Geometry check sheet. Reference: the model listing, model coordinates, mm. A direction names the side the tool comes from. Coordinates: 2 decimals unless noted, no trailing zeros. Write each loop counter-clockwise with the first axis right and the second up, starting at its lowest first coordinate (ties: lowest second). Pieces come first, ordered by that corner, then holes. Notation, with made-up numbers: (-36.5, 65) -> (8.5, 65) arc R19 cw to (8.5, 87) -> close; hole circle Ø5 at (1, 50.5). An arc over 180 degrees is marked (long way). Use a Markdown table: item, result.
```python
from build123d import *

# Parameters (mm, degrees)
F3_DEPTH = 0.2
F4_COUNT = 4
F7_DEPTH = 0.2


with BuildPart() as f1:
    # F0 (on Front) → F1 (revolve)
    with BuildSketch(Plane.XZ):
        with BuildLine():
            Line((0, 20.1388888889), (0, 0))
            Line((0, 0), (0.5555555556, 0))
            Line((0.5555555556, 0), (0.5555555556, 18.9583333333))
            Line((0.5555555556, 18.9583333333), (0.4513888889, 19.7916666667))
            ThreePointArc((0.4513888889, 19.7916666667), (0.2847433935, 20.0420414116), (0, 20.1388888889))
        make_face()
    revolve(axis=Axis((0, 0, 10.0694444444), (0, 0, 1)))

    # F2 (on Front) → F3 (join, symmetric)
    with BuildSketch(Plane.XZ):
        Polygon((0.2263558201, 19.9583333333), (-0.2263558201, 19.9583333333), (-1.8229166667, 17.9861111111), (-0.4993386243, 17.9861111111), (-2.3263888889, 15.7291666667), (2.3263888889, 15.7291666667), (0.4993386243, 17.9861111111), (1.8229166667, 17.9861111111), align=None)
        Polygon((0.5361597759, 0.0173323988), (0.5555555556, 0), (2.1875, -1.4583333333), (2.1875, 0.6597222222), (1.0069444444, 2.8125), (0.7291666667, 9.2361111111), (-0.7291666667, 9.2361111111), (-1.0069444444, 2.8125), (-2.1875, 0.6597222222), (-2.1875, -1.4583333333), (-0.5555555556, 0), (-0.5361597759, 0.0173323988), align=None)
        Polygon((-0.5555555556, 0), (0.5555555556, 0), (0.5361597759, 0.0173323988), (-0.5361597759, 0.0173323988), align=None)
    extrude(amount=F3_DEPTH, both=True)


with BuildPart() as f4_1:
    # F4: instance of F1
    add(f1.part.rotate(Axis((0, 0, 0), (0, 0, 1)), 1 * 360 / F4_COUNT))


with BuildPart() as f4_2:
    # F4: instance of F1
    add(f1.part.rotate(Axis((0, 0, 0), (0, 0, 1)), 2 * 360 / F4_COUNT))


with BuildPart() as f4_3:
    # F4: instance of F1
    add(f1.part.rotate(Axis((0, 0, 0), (0, 0, 1)), 3 * 360 / F4_COUNT))


with BuildPart() as f1_1:
    add(f1.part)

    add(f4_1.part)  # F7 merges F4_1

    add(f4_2.part)  # F7 merges F4_2

    add(f4_3.part)  # F7 merges F4_3
    # F6 (on face) → F7 (join, symmetric)
    with BuildSketch(Plane(origin=(0, 0, 0), x_dir=(0.7071067812, -0.7071067812, 0), z_dir=(-0.7071067812, -0.7071067812, 0))):
        Polygon((0.25, 15.3652419184), (-0.25, 15.3652419184), (-1.4370362347, 15), (-1.4370362347, 14.6875), (-0.25, 15.0527419184), (0.25, 15.0527419184), (1.4370362347, 14.6875), (1.4370362347, 15), align=None)
    extrude(amount=F7_DEPTH, both=True)


solid = f1_1.part
```
Item 1: Depth check by flat-ended pin: P1, Ø0.9, axis at x = 1.5, z = 17, coming from the +Y side; P2, Ø0.9, axis at y = -1.5, z = 16.5, coming from the +X side; P3, Ø1.4, axis at y = 1.5, z = 17, coming from the -X side. Enter the tip coordinate at first touch or a pass-through.
Answer block:
| item | result |
|---|---|
| P1 | stops at y = 0.2 |
| P2 | stops at x = 0.2 |
| P3 | stops at x = -0.2 |
Item 2: Section check D-D on x = 0. Record the boundary of the cut face in (y, z), then the cut area to 3 significant figures.
Answer block:
| item | result |
|---|---|
| outline | (-2.33, 15.73) -> (-0.56, 15.73) -> (-0.56, 9.24) -> (-0.73, 9.24) -> (-1.01, 2.81) -> (-2.19, 0.66) -> (-2.19, -1.46) -> (-0.56, 0) -> (0.56, 0) -> (2.19, -1.46) -> (2.19, 0.66) -> (1.01, 2.81) -> (0.73, 9.24) -> (0.56, 9.24) -> (0.56, 15.73) -> (2.33, 15.73) -> (0.56, 17.92) -> (0.56, 17.99) -> (1.82, 17.99) -> (0.47, 19.66) -> (0.45, 19.79) arc R0.47 ccw to (-0.45, 19.79) -> (-0.47, 19.66) -> (-1.82, 17.99) -> (-0.56, 17.99) -> (-0.56, 17.92) -> close |
| area | 41.1 mm^2 |
Item 3: Thickness scan on L1, parallel to Y at x = -1, z = 0.25; L2, parallel to Z at x = -1.9, y = 0.05. Record the ranges inside material, lowest first. Write a range as [from, to].
Answer block:
| item | result |
|---|---|
| L1 | y = [-0.2, 0.2] |
| L2 | z = [-1.2, 1.18], [15.73, 16.26] |
Item 4: Section check B-B on y = 1.45. Record the boundary of the cut face in (x, z), then the cut area to 3 significant figures.
Answer block:
| item | result |
|---|---|
| outline | (-0.2, -0.8) -> (0.2, -0.8) -> (0.2, 2) -> (-0.2, 2) -> close; (-0.2, 15.73) -> (0.2, 15.73) -> (0.2, 16.81) -> (-0.2, 16.81) -> close; (-0.2, 17.99) -> (0.2, 17.99) -> (0.2, 18.45) -> (-0.2, 18.45) -> close |
| area | 1.74 mm^2 |
Item 5: Tool access check on faces 1 (the flat face through (-1.383, -0.003, -0.739)), 2 (the flat face through (1.605, -0.003, 1.721)), 3 (the flat face through (0.8, 0.2, 2.8)). Record the directions out of +Z, -Z, +X, -X, +Y, -Y that give a thin tool (end or side, any length) a straight path to the whole face; none if there is none.
Answer block:
| item | result |
|---|---|
| face 1 | -Z, +Y, -Y |
| face 2 | +X, +Y, -Y |
| face 3 | +Z, -Z, +X, +Y |
Item 6: Section check A-A on x = 1.55. Record the boundary of the cut face in (y, z).
Answer block:
| item | result |
|---|---|
| outline | (-0.2, -0.89) -> (0.2, -0.89) -> (0.2, 1.82) -> (-0.2, 1.82) -> close; (-0.2, 15.73) -> (0.2, 15.73) -> (0.2, 16.69) -> (-0.2, 16.69) -> close; (-0.2, 17.99) -> (0.2, 17.99) -> (0.2, 18.32) -> (-0.2, 18.32) -> close |
Item 7: Mould release check, pull along Z, two halves, no side actions. Record for faces 4 (the flat face through (-0.698, 0.694, 14.827)), 5 (the flat face through (-0.2, -1, 2)), 6 (the flat face through (-0.003, 1.435, 16.83)): +Z half, -Z half, draft (parallel to the pull), parting line (faces both ways), or undercut.
Answer block:
| item | result |
|---|---|
| face 4 | -Z half |
| face 5 | draft |
| face 6 | undercut |
Item 8: Section check C-C on z = 0.25. Record the boundary of the cut face in (x, y).
Answer block:
| item | result |
|---|---|
| outline | (-2.19, -0.2) -> (-0.52, -0.2) arc R0.56 ccw to (-0.2, -0.52) -> (-0.2, -2.19) -> (0.2, -2.19) -> (0.2, -0.52) arc R0.56 ccw to (0.52, -0.2) -> (2.19, -0.2) -> (2.19, 0.2) -> (0.52, 0.2) arc R0.56 ccw to (0.2, 0.52) -> (0.2, 2.19) -> (-0.2, 2.19) -> (-0.2, 0.52) arc R0.56 ccw to (-0.52, 0.2) -> (-2.19, 0.2) -> close |
